The drawing under review shows one solid part. Ordinate dimensions are in mm from its lowest x, y, z. Round coordinates to 2 decimals unless told otherwise and drop trailing zeros. Order: outer loops, then holes, each group sorted by start corner. A loop starts at its lowest first (then second) coordinate and runs counter-clockwise, first axis right, second up. Notation, with made-up numbers: M 32.5,-0.5 L 77.5,-0.5 A27 cw 77.5,28.5 Z; hole C 68,-37.5 d5. An arc over 180 degrees is marked long. Answer as a JSON object with one key per item and string values. Group by question number.
1) Insertion check: pin 1 Ø1.5 at (x, y) = (226, 3) entering from +Z; pin 2 Ø1 at (x, y) = (93, 4) entering from +Z. Each pin has a flat end and moves straight along its axis. Give the tip position at first contact, or say it passes through.
2) Consider section D-D, the plane x = 246.5. Write out the cut boundary in (y, z).
3) Consider section B-B, the plane y = 3. Write out the cut boundary in (x, z).
4) To check wall thickness, follow line 1 (X direction, y = 0.5, z = 34); line 2 (X direction, y = 6.75, z = 33); line 3 (Z direction, x = 150.5, y = 3). State the ranges of each line that lie inside material, in increasing order.
5) Consider section A-A, the plane z = 30. Write out the cut boundary in (x, y), then the cut area to 3 significant figures.
6) Consider section C-C, the plane x = 30. Write out the cut boundary in (y, z).
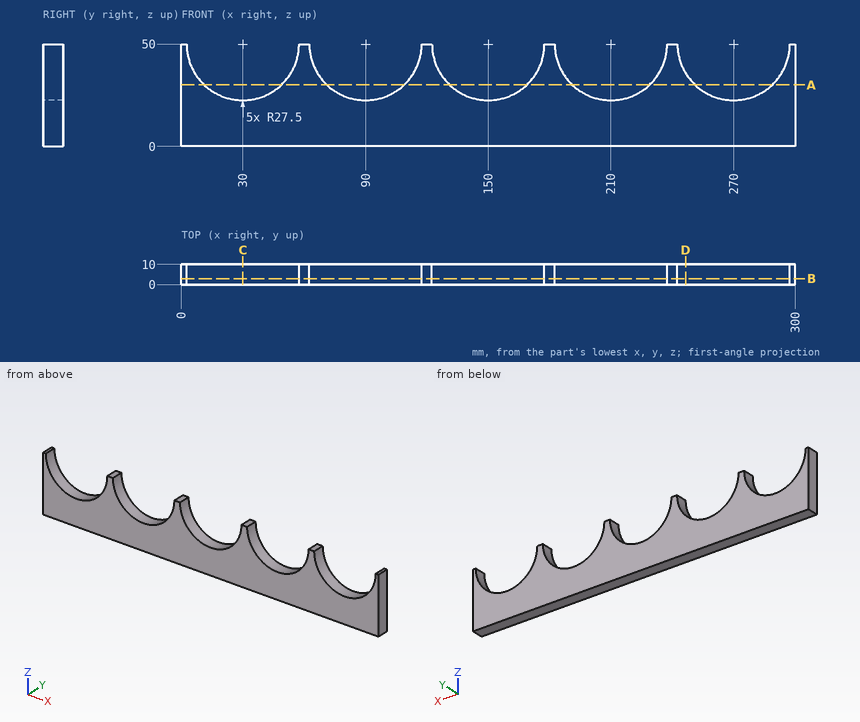
Results list:
{
 "1": {"pin 1": "z = 28.19", "pin 2": "z = 22.72"},
 "2": {"outline": "M 0,0 L 10,0 L 10,35.72 L 0,35.72 Z"},
 "3": {"outline": "M 0,0 L 300,0 L 300,50 L 297.5,50 A27.5 cw 242.5,50 L 237.5,50 A27.5 cw 182.5,50 L 177.5,50 A27.5 cw 122.5,50 L 117.5,50 A27.5 cw 62.5,50 L 57.5,50 A27.5 cw 2.5,50 L 0,50 Z"},
 "4": {"line 1": "0 to 7.63, 52.37 to 67.63, 112.37 to 127.63, 172.37 to 187.63, 232.37 to 247.63, 292.37 to 300", "line 2": "0 to 8.38, 51.62 to 68.38, 111.62 to 128.38, 171.62 to 188.38, 231.62 to 248.38, 291.62 to 300", "line 3": "0 to 22.5"},
 "5": {"outline": "M 0,0 L 11.13,0 L 11.13,10 L 0,10 Z; M 48.87,0 L 71.13,0 L 71.13,10 L 48.87,10 Z; M 108.87,0 L 131.13,0 L 131.13,10 L 108.87,10 Z; M 168.87,0 L 191.13,0 L 191.13,10 L 168.87,10 Z; M 228.87,0 L 251.13,0 L 251.13,10 L 228.87,10 Z; M 288.87,0 L 300,0 L 300,10 L 288.87,10 Z", "area": "1,110 mm^2"},
 "6": {"outline": "M 0,0 L 10,0 L 10,22.5 L 0,22.5 Z"}
}
